Job drawing, mm, ordinate dimensions from the low corner. One solid piece. Coordinates: 2 decimals unless noted, no trailing zeros. Order: outer loops, then holes, each group sorted by start corner. A loop starts at its lowest first (then second) coordinate and runs counter-clockwise, first axis right, second up. Notation, with made-up numbers: (71.5, 45) - (84.5, 45) arc R20 cw to (84.5, 82) - close; hole circle Ø3 at (64, -30). An arc over 180 degrees is marked (long way). Use a Markdown table: item, result. Add a question column.
1) Saw through at C-C on z = 43. List the corners of the cut face in (x, y).
2) Saw through at A-A on z = 56. List the corners of the cut face in (x, y), then the cut area to 3 significant figures.
3) Saw through at B-B on y = 45. List the corners of the cut face in (x, z), then the cut area to 3 significant figures.
4) Wall check: L1, parallel to X at y = 16, z = 21. Give the ranges that are in metal, low to high. Write a range as [from, to].
5) Drop a flat-ended pin along its axis: P1, Ø18, axis at y = 39.5, z = 28, coming from the -X side. Give the stop position or say it passes through.
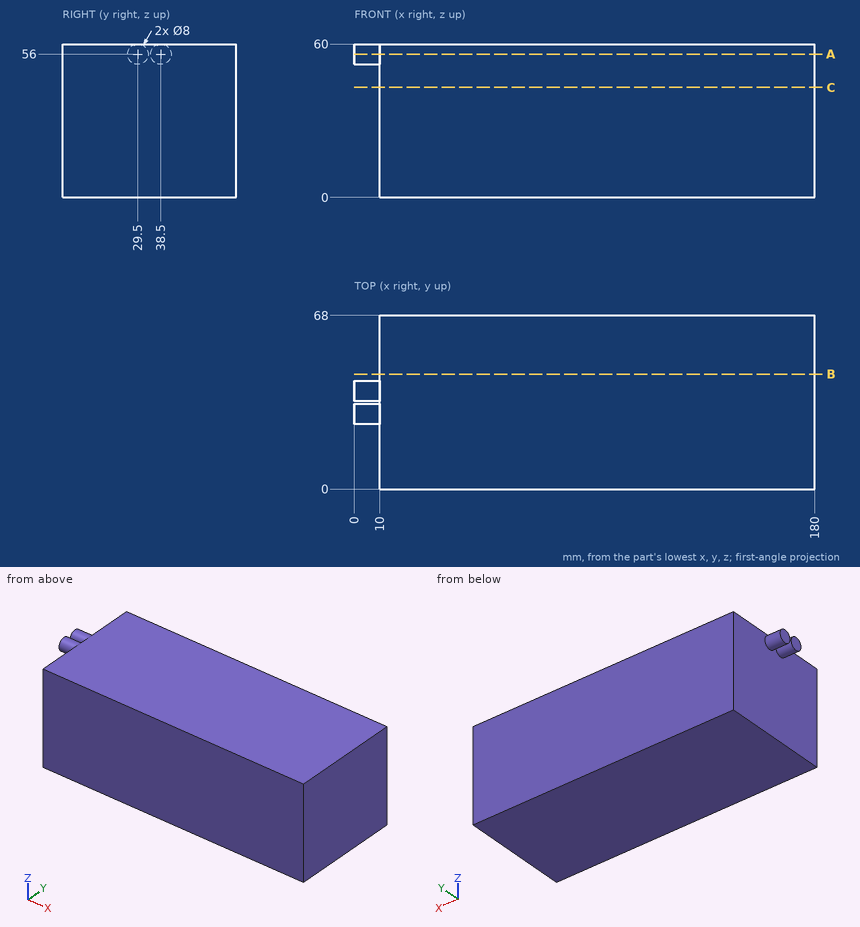
Results are:
| question | item | result |
|---|---|---|
| 1 | outline | (10, 0) - (180, 0) - (180, 68) - (10, 68) - close |
| 2 | outline | (0, 25.5) - (10, 25.5) - (10, 0) - (180, 0) - (180, 68) - (10, 68) - (10, 42.5) - (0, 42.5) - (0, 34.5) - (10, 34.5) - (10, 33.5) - (0, 33.5) - close |
| 2 | area | 11,700 mm2 |
| 3 | outline | (10, 0) - (180, 0) - (180, 60) - (10, 60) - close |
| 3 | area | 10,200 mm2 |
| 4 | L1 | [10, 180] |
| 5 | P1 | x = 10 |
